from build123d import *

# Parameters (mm, degrees)
SKETCH1_W               = 4.671
SKETCH1_H               = 15.746
SKETCH1_W_2             = 7
SKETCH1_H_2             = 2
SKETCH1_W_3             = 22.4
SKETCH1_H_3             = 3.746
BOSS_EXTRUDE1_DEPTH     = 13
CUT_EXTRUDE1_DEPTH      = 60.119451433
CUT_EXTRUDE1_DEPTH_BACK = 60.119451433
SKETCH2_R               = 1.55


with BuildPart() as part:
    # Sketch1 → Boss-Extrude1 (new body)
    with BuildSketch(Plane.XY):
        with Locations((-46.693035151, 12.873)):
            Rectangle(SKETCH1_W, SKETCH1_H)
        with Locations((-52.528535151, 6)):
            Rectangle(SKETCH1_W_2, SKETCH1_H_2)
        with Locations((-33.157535151, 18.873)):
            Rectangle(SKETCH1_W_3, SKETCH1_H_3)
        Polygon((-21.957535151, 20.746), (-21.957535151, 17), (-21.957535151, 5.074394878), (-17.106930028, 5.074394878), (-17.106930028, 7.074394878), (-17.106930028, 20.746), align=None)
        with Locations((-13.606930028, 6.074394878)):
            Rectangle(SKETCH1_W_2, SKETCH1_H_2)
    extrude(amount=BOSS_EXTRUDE1_DEPTH)

    # Sketch2 → Cut-Extrude1 (cut, two sides: drawn at the far end of the back side and taken through both)
    with BuildSketch(Plane(origin=(0, 7.074394878, 0), x_dir=(1, 0, 0), z_dir=(0, 1, 0)).offset(-CUT_EXTRUDE1_DEPTH_BACK)):
        with Locations(Location((-13.606930028, -9.75, 0), (0, 0, 270))):
            Circle(SKETCH2_R)
        with Locations(Location((-13.606930028, -3.25, 0), (0, 0, 270))):
            Circle(SKETCH2_R)
        with Locations(Location((-52.528535151, -3.25, 0), (0, 0, 270))):
            Circle(SKETCH2_R)
        with Locations((-52.528535151, -9.75)):
            Circle(SKETCH2_R)
    extrude(amount=CUT_EXTRUDE1_DEPTH + CUT_EXTRUDE1_DEPTH_BACK, mode=Mode.SUBTRACT)


solid = part.part
Verification items for the finished model (mm, model axes). A direction names the side the tool comes from. Round coordinates to 2 decimals unless told otherwise and drop trailing zeros. Order: outer loops, then holes, each group sorted by start corner. A loop starts at its lowest first (then second) coordinate and runs counter-clockwise, first axis right, second up.
1. Thickness scan on L1, parallel to X at y = 12, z = 5.5; L2, parallel to X at y = 5.85, z = 3.25; L3, parallel to Y at x = -43, z = 3.25. Record the ranges inside material, lowest first.
Final values:
L1: x = -49.03 to -44.36, -21.96 to -17.11
L2: x = -56.03 to -54.08, -50.98 to -44.36, -21.96 to -15.16, -12.06 to -10.11
L3: y = 17 to 20.75
2. Release check for a two-part mould opening along X. For faces 1 (the flat face through (-49.029, 14, 6)), 2 (the flat face through (-17.107, 14, 6)), 3 (the flat face through (-50, 5, 6)), 4 (the flat face through (-33, 17, 6)) record: +X half, -X half, draft (parallel to the pull), parting line (faces both ways), or undercut.
Final values:
face 1: -X half
face 2: +X half
face 3: draft
face 4: undercut
3. Section check D-D on y = 17.5. Record the cut outline in (x, z), then the cut area to 3 significant figures.
Final values:
outline: (-49.03, 0) - (-17.11, 0) - (-17.11, 13) - (-49.03, 13) - close
area: 415 mm2
4. Access from +Z, -Z, +X, -X, +Y, -Y to the whole of each face (thin tool, end or side, straight path). Record for faces 5 (the flat face through (-16, 5.074, 6)), 6 (the flat face through (-44.358, 11, 6)), 7 (the flat face through (-53, 7, 6)), 8 (the flat face through (-56.029, 6, 6)), 9 (the flat face through (-14, 7.074, 6)).
Final values:
face 5: +Z, -Z, +X, -Y
face 6: +Z, -Z, -Y
face 7: +Z, -Z, -X, +Y
face 8: +Z, -Z, -X, +Y, -Y
face 9: +Z, -Z, +X, +Y
5. Section check B-B on z = 3.25. Record the cut outline in (x, y).
Final values:
outline: (-56.03, 5) - (-54.08, 5) - (-54.08, 7) - (-56.03, 7) - close; (-50.98, 5) - (-44.36, 5) - (-44.36, 17) - (-21.96, 17) - (-21.96, 5.07) - (-15.16, 5.07) - (-15.16, 7.07) - (-17.11, 7.07) - (-17.11, 20.75) - (-49.03, 20.75) - (-49.03, 7) - (-50.98, 7) - close; (-12.06, 5.07) - (-10.11, 5.07) - (-10.11, 7.07) - (-12.06, 7.07) - close
6. Go/stop test with flat-tipped pins: P1, Ø4, axis at y = 15, z = 3.5, coming from the +X side; P2, Ø6, axis at y = 12.5, z = 9.5, coming from the -X side; P3, Ø4, axis at x = -13.61, z = 9.75, coming from the +Y side; P4, Ø3, axis at x = -52.53, z = 9.75, coming from the -Y side. Record where each tip stops, or that it passes through.
Final values:
P1: stops at x = -17.11
P2: stops at x = -49.03
P3: stops at y = 7.07
P4: passes through
7. Section check C-C on x = -16.5. Record the cut outline in (y, z).
Final values:
outline: (5.07, 0) - (7.07, 0) - (7.07, 13) - (5.07, 13) - close
8. Section check A-A on y = 9.25. Record the cut outline in (x, z).
Final values:
outline: (-49.03, 0) - (-44.36, 0) - (-44.36, 13) - (-49.03, 13) - close; (-21.96, 0) - (-17.11, 0) - (-17.11, 13) - (-21.96, 13) - close
